Autodesk Inventor part; units mm, degrees
ref_plane "YZ Plane" through (0, 0, 0) normal (1, 0, 0) x (0, 1, 0)
ref_plane "XZ Plane" through (0, 0, 0) normal (0, 1, 0) x (-1, 0, 0)
ref_plane "XY Plane" through (0, 0, 0) normal (0, 0, 1) x (1, 0, 0)
sketch "Эскиз1" plane through (0, 0, 0) normal (0, 1, 0) x (-1, 0, 0)
  line L0 (102, 151) -> (42, 151)
  line L1 (42, -149) -> (102, -149)
  line L2 (102, -149) -> (102, 151)
  line L3 (102, 151) -> (42, 151)
  line L4 (42, 151) -> (42, 176)
  line L5 (42, 176) -> (102, 176)
  line L6 (102, 176) -> (102, 151)
  line L7 (102, -149) -> (42, -149)
  line L8 (42, -149) -> (42, -124)
  line L9 (42, -124) -> (102, -124)
  line L10 (102, -124) -> (102, -149)
  line L11 (42, 176) -> (42, -124)
  line L12 (42, 176) -> (17, 176)
  line L13 (17, 176) -> (17, -149)
  line L14 (17, -149) -> (42, -149)
  line L15 (42, -149) -> (42, 176)
  point P0 (0, 0)
  point P1 (42, 151)
  dimension "d0" = 300
  dimension "d1" = 60
  dimension "d2" = 25
  dimension "d3" = 25
  dimension "d5" = 25
  dimension "d33" = 25
extrude "Выдавливание1" add sketch "Эскиз1" along normal blind 190 contours L0 L4 L5 L6 | L11 L8 L14 L13 L12 L4 | L2 L1 L8 L9
sketch "Эскиз2" plane through (-17, 0, 176) normal (1, 0, 0) x (0, 0, -1)
  line L0 (0, 0) -> (325, 0)
  line L1 (325, 0) -> (325, 190)
  line L2 (0, 190) -> (325, 190)
  line L3 (0, 0) -> (0, 190)
  line L4 (-98, 158) -> (488, 158)
  line L5 (488, 158) -> (488, 32)
  line L6 (488, 32) -> (-98, 32)
  line L7 (-98, 32) -> (-98, 158)
  point P0 (176, 0)
  point P1 (325, 32)
  point P2 (0, 32)
  point P3 (0, 158)
  point P4 (325, 158)
  dimension "d8" = 32
  dimension "d9" = 32
extrude "Выдавливание2" cut sketch "Эскиз2" against normal blind 0.5 contours L3 L6 L1 L0 | L3 L2 L1 L4
sketch "Эскиз4" plane through (-102, 0, -149) normal (0, 0, -1) x (-1, 0, 0)
  line L0 (-85, 32) -> (-84.5, 32)
  line L1 (-84.5, 32) -> (-84.5, 0)
  line L2 (-84.5, 0) -> (0, 0)
  line L3 (0, 0) -> (0, 190)
  line L4 (-84.5, 190) -> (0, 190)
  line L5 (-84.5, 190) -> (-84.5, 158)
  line L6 (-84.5, 158) -> (-85, 158)
  line L7 (-85, 32) -> (-85, 158)
  line L8 (-92, 195) -> (-65, 195)
  line L9 (-65, 195) -> (-65, -10)
  line L10 (-65, -10) -> (-92, -10)
  line L11 (-92, -10) -> (-92, 195)
  point P0 (-102, 0)
  point P1 (-65, 0)
  point P2 (-65, 190)
  dimension "d12" = 20
extrude "Выдавливание3" add sketch "Эскиз4" along normal blind 70 contours L7 L6 L5 L4 L9 L2 L1 L0
sketch "Эскиз5" plane through (-17, 32, 176) normal (1, 0, 0) x (0, 0, -1)
  line L0 (0, 0) -> (395, 0)
  line L1 (395, 126) -> (395, 0)
  line L2 (0, 126) -> (395, 126)
  line L3 (0, 0) -> (0, 126)
  line L4 (-43, 93) -> (474, 93)
  line L5 (474, 93) -> (474, 33)
  line L6 (474, 33) -> (-43, 33)
  line L7 (-43, 33) -> (-43, 93)
  point P0 (176, -32)
  dimension "d15" = 33
  dimension "d16" = 33
extrude "Выдавливание4" cut sketch "Эскиз5" against normal blind 10 contours L6 L7 L4 L3 | L3 L4 L1 L6 | L1 L4 L5 L6
sketch "Эскиз6" plane through (-102, 0, -149) normal (-1, 0, 0) x (0, 0, 1)
  line L0 (0, 0) -> (25, 0)
  line L1 (25, 0) -> (25, 190)
  line L2 (0, 190) -> (25, 190)
  line L3 (0, 0) -> (0, 190)
  line L4 (300, 0) -> (325, 0)
  line L5 (325, 0) -> (325, 190)
  line L6 (300, 190) -> (325, 190)
  line L7 (300, 0) -> (300, 190)
  line L8 (325, 190) -> (-70, 190)
  line L9 (300, 0) -> (325, 0)
  line L10 (325, 190) -> (312.5, 190)
  line L11 (312.5, 190) -> (312.5, 0)
  line L12 (312.5, 0) -> (325, 0)
  line L13 (325, 0) -> (325, 190)
  line L14 (0, 190) -> (25, 190)
  line L15 (0, 0) -> (25, 0)
  line L16 (0, 190) -> (12.5, 190)
  line L17 (12.5, 190) -> (12.5, 0)
  line L18 (12.5, 0) -> (0, 0)
  line L19 (0, 0) -> (0, 190)
  line L20 (347, 70) -> (-28, 70)
  line L21 (-28, 70) -> (-28, 120)
  line L22 (-28, 120) -> (347, 120)
  line L23 (347, 120) -> (347, 70)
  point P0 (149, 0)
  point P1 (12.5, 0)
  point P2 (12.5, 190)
  point P3 (12.5, 70)
  point P4 (0, 70)
  point P5 (0, 120)
  point P6 (12.5, 120)
  point P7 (325, 70)
  point P8 (312.5, 70)
  point P9 (312.5, 120)
  point P10 (325, 120)
  dimension "d21" = 70
  dimension "d22" = 70
extrude "Выдавливание5" cut sketch "Эскиз6" against normal blind 15 contours L3 L20 L17 L0 | L3 L2 L17 L22 | L20 L5 L4 L11 | L11 L6 L5 L22
fillet "Сопряжение1" radius 6 4 edges at (-94.5, 70, -136.5) (-94.5, 120, -136.5) (-94.5, 120, 163.5) (-94.5, 70, 163.5)
sketch "Эскиз8" plane through (-17, 158, 176) normal (1, 0, 0) x (0, 0, -1)
  line L0 (376, -40) -> (389, -40)
  line L1 (389, -40) -> (389, -86)
  line L2 (389, -86) -> (376, -86)
  line L3 (376, -86) -> (376, -40)
  line L4 (395, -33) -> (395, -93)
  circle A0 centre (389, -40) radius 3
  circle A1 centre (389, -86) radius 3
  circle A2 centre (376, -40) radius 3
  circle A3 centre (376, -86) radius 3
  point P0 (176, -158)
  dimension "d24" = 6
  dimension "d25" = 46
  dimension "d26" = 13
extrude "Выдавливание6" cut sketch "Эскиз8" against normal blind 100 contours L3 A2 L0 | L0 A2 L3 | A0 L1 L0 | L0 L1 A0 | A3 L2 L3 | L3 L2 A3 | A1 L2 L1 | L1 L2 A1
sketch "Эскиз9" plane through (-102, 0, -219) normal (0, 0, -1) x (-1, 0, 0)
  line L0 (-84.5, 190) -> (-84.5, 158)
  line L1 (-65, 0) -> (-15, 0)
  line L2 (-84.5, 190) -> (-65, 190)
  line L3 (-65, 190) -> (-65, 0)
  line L4 (-65, 0) -> (-84.5, 0)
  line L5 (-84.5, 0) -> (-84.5, 190)
  point P0 (-102, 0)
  point P1 (-84.5, 158)
extrude "Выдавливание7" add sketch "Эскиз9" along normal blind 10
sketch "Эскиз10" plane through (-42, 0, -124) normal (-1, 0, 0) x (0, 0, 1)
  line L0 (159.1033, 24) -> (108.1033, 24)
  line L1 (159.1033, 63) -> (159.1033, 24)
  line L2 (108.1033, 63) -> (159.1033, 63)
  line L3 (108.1033, 24) -> (108.1033, 63)
  circle A0 centre (153.6033, 31.5) radius 2.75
  circle A1 centre (113.6033, 31.5) radius 2.75
  circle A2 centre (113.6033, 55.5) radius 2.75
  circle A3 centre (153.6033, 55.5) radius 2.75
  line L4 (158.6033, 104) -> (159.6033, 104)
  line L5 (159.1033, 104) -> (159.1033, 63)
  line L6 (159.1033, 104) -> (108.1033, 104)
  line L7 (159.1033, 143) -> (159.1033, 104)
  line L8 (108.1033, 143) -> (159.1033, 143)
  line L9 (108.1033, 104) -> (108.1033, 143)
  circle A4 centre (153.6033, 111.5) radius 2.75
  circle A5 centre (113.6033, 111.5) radius 2.75
  circle A6 centre (113.6033, 135.5) radius 2.75
  circle A7 centre (153.6033, 135.5) radius 2.75
  line L10 (275, 0) -> (275, 190)
  line L11 (275, 26) -> (165, 26)
  line L12 (165, 26) -> (165, 46)
  line L13 (165, 46) -> (275, 46)
  line L14 (275, 46) -> (275, 26)
  line L15 (165, 26) -> (163, 26)
  line L16 (164.1033, 26) -> (164.1033, 24)
  point P0 (124, 0)
  point P1 (133.6033, 23.5)
  point P2 (133.6033, 103.5)
extrude "Выдавливание8" cut sketch "Эскиз10" against normal blind 33 contours A0 | A1 | A2 | A3 | A4 | A5 | A6 | A7
sketch "Sketch11" plane through (0, 190, 0) normal (0, 1, 0) x (1, 0, 0)
  line L0 (-42, -151) -> (-102, -151)
  line L1 (-102, -151) -> (-42, -151)
  line L2 (-42, -151) -> (-42, -151.5)
  line L3 (-42, -151.5) -> (-102, -151.5)
  line L4 (-102, -151.5) -> (-102, -151)
  line L5 (-102, 124) -> (-42, 124)
  line L6 (-42, 124) -> (-42, 124.5)
  line L7 (-42, 124.5) -> (-102, 124.5)
  line L8 (-102, 124.5) -> (-102, 124)
  line L9 (-17.5, -176) -> (-17.5, 229)
  point P0 (0, 0)
  dimension "d34" = 24.5
  dimension "d35" = 24.5
  dimension "d36" = 0.5
  dimension "d37" = 0.5
extrude "Extrusion9" cut sketch "Sketch11" against normal blind 200
sketch "Sketch12" plane through (-42, 0, 151.5) normal (-1, 0, 0) x (0, 0, 1)
  line L0 (-276, 190) -> (-276, 0)
  line L1 (-276, 80) -> (-264, 80)
  line L2 (-264, 80) -> (-264, 110)
  line L3 (-264, 110) -> (-276, 110)
  line L4 (-276, 110) -> (-276, 80)
  line L5 (0, 190) -> (0, 0)
  line L6 (0, 80) -> (-12, 80)
  line L7 (-12, 80) -> (-12, 110)
  line L8 (-12, 110) -> (0, 110)
  line L9 (0, 110) -> (0, 80)
  line L10 (-276, 190) -> (0, 190)
  line L11 (0, 0) -> (-276, 0)
  point P0 (-151.5, 0)
  point P1 (0, 110)
  dimension "d40" = 80
  dimension "d41" = 80
  dimension "d42" = 80
  dimension "d43" = 80
  dimension "d46" = 12
  dimension "d47" = 12
extrude "Extrusion10" add sketch "Sketch12" along normal blind 40 contours L3 L2 L1 L0 | L5 L6 L7 L8
properties part number "KaretkaY"
Input: part model. Units: mm. Frame: model coordinates. A direction names the side the tool comes from. Round coordinates to 2 decimals unless told otherwise and drop trailing zeros. Order: outer loops, then holes, each group sorted by start corner. A loop starts at its lowest first (then second) coordinate and runs counter-clockwise, first axis right, second up. Notation, with made-up numbers: (44, -9) - (74, -9) arc R17 ccw to (74, -4) - close; hole circle Ø3 at (-29, 40). An arc over 180 degrees is marked (long way). One line per question, with ' | ' between items. Start each with the question number.
1) Cut plane A-A, the plane x = -70.5. Return the cut outline in (y, z), then the cut area to 3 significant figures.
2) Set-up query: faces 4 (the flat face through (-27, 95, -19)), 5 (the flat face through (-62, 80, 146)), 6 (the flat face through (-82, 95, -119)), 7 (the flat face through (-87, 155, -143)). Return all of +Z, -Z, +X, -X, +Y, -Y with unobstructed straight access to the full face (end or side cutting, diameter ignored); none if empty.
3) Cut plane B-B, the plane z = -76. Return the cut outline in (x, y), then the cut area to 3 significant figures.
4) Cut plane C-C, the plane y = 166. Return the cut outline in (x, z).
5) Pull-direction query (Z, two-part tool) for faces 1 (the flat face through (-17.5, 159, -56)), 2 (the flat face through (-95, 158, -136.5)), 3 (the flat face through (-62, 110, -118)); classes: +Z half, -Z half, draft (parallel to the pull), parting line (faces both ways), or undercut.
6) Contact query for flat-ended pins moving along their axis: P1, Ø3.5, axis at y = 118, z = -200, coming from the -X side; P2, Ø7.5, axis at x = -91.5, y = 35.5, coming from the -Z side; P3, Ø6, axis at y = 146, z = 170, coming from the -X side; P4, Ø2, axis at x = -70.5, y = 107.5, coming from the -Z side. Output: stop coordinate, or through.
7) Ray query, probe 1 along Z at (x, y) = (-22, 135); probe 2 along Y at (x, z) = (-29.75, -213); probe 3 along Z at (x, y) = (-84.5, 137). Return the intervals inside material, ascending.
Worked out:
1) outline: (0, -149) - (190, -149) - (190, -124.5) - (110, -124.5) - (110, -112.5) - (80, -112.5) - (80, -124.5) - (0, -124.5) - close; (0, 151.5) - (80, 151.5) - (80, 139.5) - (110, 139.5) - (110, 151.5) - (190, 151.5) - (190, 176) - (0, 176) - close | area: 10,000 mm^2
2) face 4: +Z, +X | face 5: -X, -Y | face 6: -X, +Y, -Y | face 7: -Z, -X, +Y
3) outline: (-42, 0) - (-17.5, 0) - (-17.5, 32) - (-17, 32) - (-17, 65) - (-27, 65) - (-27, 125) - (-17, 125) - (-17, 158) - (-17.5, 158) - (-17.5, 190) - (-42, 190) - close | area: 4,120 mm^2
4) outline: (-102, -136.5) - (-87, -136.5) - (-87, -149) - (-37, -149) - (-37, -229) - (-17.5, -229) - (-17.5, 176) - (-87, 176) - (-87, 163.5) - (-102, 163.5) - (-102, 151.5) - (-42, 151.5) - (-42, -124.5) - (-102, -124.5) - close
5) face 1: draft | face 2: -Z half | face 3: undercut
6) P1: passes through | P2: stops at z = -136.5 | P3: stops at x = -87 | P4: stops at z = -149
7) probe 1: z = -229 to -13.1, -7.69 to 26.9, 32.31 to 176 | probe 2: y = 0 to 69, 75 to 115, 121 to 190 | probe 3: z = -149 to -124.5, 151.5 to 176
